from build123d import *

# Parameters (mm, degrees)
SKETCH1_R      = 12.7
EXTRUDE2_DEPTH = 25.4


with BuildPart() as part:
    # Sketch1 → Extrude2 (new body)
    with BuildSketch(Plane(origin=(0, 0, 0), x_dir=(1, 0, 0), z_dir=(0, 1, 0))):
        with BuildLine():
            Line((-31.75, 21.298547486), (-31.75, -21.298547486))
            ThreePointArc((-31.75, -21.298547486), (-30.643460801, -26.483300775), (-27.516666667, -30.76456859))
            ThreePointArc((-27.516666667, -30.76456859), (0, -41.275), (27.516666667, -30.76456859))
            ThreePointArc((27.516666667, -30.76456859), (30.643460801, -26.483300775), (31.75, -21.298547486))
            Line((31.75, -21.298547486), (31.75, 21.298547486))
            ThreePointArc((31.75, 21.298547486), (30.643460801, 26.483300775), (27.516666667, 30.76456859))
            ThreePointArc((27.516666667, 30.76456859), (0, 41.275), (-27.516666667, 30.76456859))
            ThreePointArc((-27.516666667, 30.76456859), (-30.643460801, 26.483300775), (-31.75, 21.298547486))
        make_face()
        with Locations(Location((0, 0, 0), (0, 0, 270))):
            Circle(SKETCH1_R, mode=Mode.SUBTRACT)
    extrude(amount=EXTRUDE2_DEPTH)


solid = part.part
Design review of the part built by this model. Coordinates are the model's own, in mm. Round coordinates to 2 decimals unless told otherwise and drop trailing zeros. Write each loop counter-clockwise with the first axis right and the second up, starting at its lowest first coordinate (ties: lowest second). Pieces come first, ordered by that corner, then holes. Notation, with made-up numbers: (-14.5, 47) - (28.5, 47) arc R19 ccw to (28.5, 62) - close; hole circle Ø1 at (71.5, 1). An arc over 180 degrees is marked (long way). Return JSON: item names as keys, results as strings. Group by question number.
Item 1: We need section A-A on z = 0. Write out the cut boundary in (x, y), and give its area (3 significant figures).
Item 2: We need section C-C on y = 18.75. Write out the cut boundary in (x, z) (3 decimals), and give its area (3 significant figures).
Item 3: The part is to be moulded in two halves that separate along X. For faces 1 (the face through (-7.7, 12.5, -10.1)), 2 (the face through (30.674, 12.522, -26.415)), 3 (the face through (-30.613, 12.522, -26.551)), say which applies: pulls with the +X half, pulls with the -X half, needs draft (parallel to the pull), parting line crosses it, or undercut.
Item 4: Insertion check: P1, Ø2, axis at y = 19.5, z = -33, coming from the +X side; P2, Ø4, axis at x = 25.5, y = 22, coming from the -Z side; P3, Ø10, axis at x = 23, y = 15.5, coming from the -Z side. Each pin has a flat end and moves straight along its axis. Give the tip position at first contact, or say it passes through.
Item 5: For probe 1 along X at (y, z) = (7.25, 0); probe 2 along Z at (x, y) = (-11.5, 15.5); probe 3 along Z at (x, y) = (-8, 5.5), list the stretches that pass through material, from the lowest coordinate up. Write a range as [from, to].
Item 6: We need section B-B on x = 0. Write out the cut boundary in (y, z) (3 decimals), and give its area (3 significant figures).
Item 7: We need section D-D on x = 20.5. Write out the cut boundary in (y, z).
Model answer:
{
 "1": {"outline": "(-31.75, 0) - (-12.7, 0) - (-12.7, 25.4) - (-31.75, 25.4) - close; (12.7, 0) - (31.75, 0) - (31.75, 25.4) - (12.7, 25.4) - close", "area": "968 mm²"},
 "2": {"outline": "(-31.75, -21.299) arc R12.7 ccw to (-27.517, -30.765) arc R41.275 ccw to (27.517, -30.765) arc R12.7 ccw to (31.75, -21.299) - (31.75, 21.299) arc R12.7 ccw to (27.517, 30.765) arc R41.275 ccw to (-27.517, 30.765) arc R12.7 ccw to (-31.75, 21.299) - close; hole circle Ø25.4 at (0, 0)", "area": "4,140 mm²"},
 "3": {"face 1": "undercut", "face 2": "pulls with the +X half", "face 3": "pulls with the -X half"},
 "4": {"P1": "stops at x = 26.07", "P2": "stops at z = -33.93", "P3": "stops at z = -37.14"},
 "5": {"probe 1": "x = [-31.75, -12.7], [12.7, 31.75]", "probe 2": "z = [-39.64, -5.39], [5.39, 39.64]", "probe 3": "z = [-40.49, -9.86], [9.86, 40.49]"},
 "6": {"outline": "(0, -41.275) - (25.4, -41.275) - (25.4, -12.7) - (0, -12.7) - close; (0, 12.7) - (25.4, 12.7) - (25.4, 41.275) - (0, 41.275) - close", "area": "1,450 mm²"},
 "7": {"outline": "(0, -35.82) - (25.4, -35.82) - (25.4, 35.82) - (0, 35.82) - close"}
}
